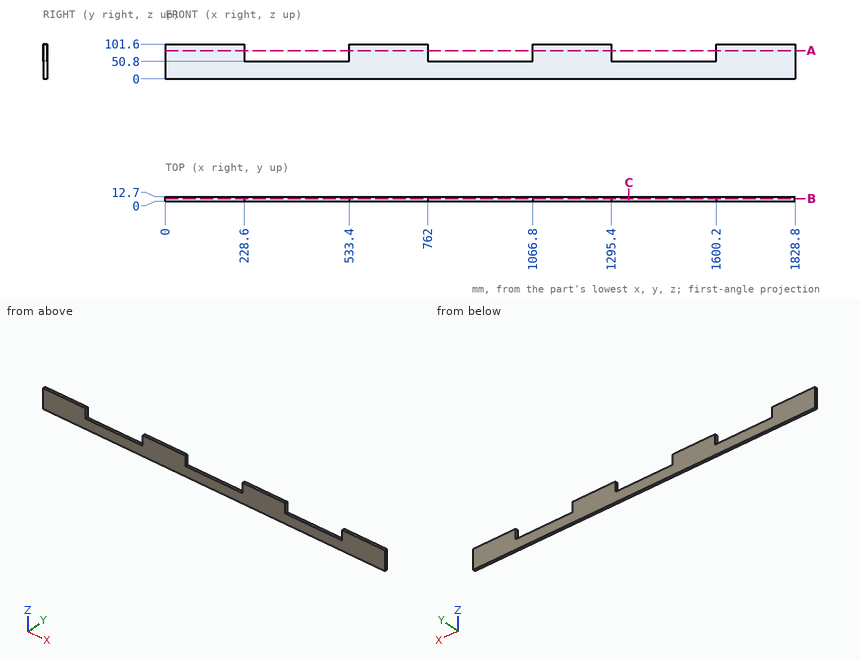
Could you check a few things on this drawing? It's one solid part, dimensions in mm from its lowest x, y, z. Give positions to 0.01 mm unless a question says otherwise; leave off trailing zeros. Write each loop counter-clockwise with the first axis right and the second up, starting at its lowest first coordinate (ties: lowest second). Pieces come first, ordered by that corner, then holes. Notation, with made-up numbers: (8.5, 38) -> (12.5, 38) arc R22 ccw to (12.5, 51) -> close; hole circle Ø5 at (37, 2). An arc over 180 degrees is marked (long way). Answer as CSV lines item,"result". Start each with the question number.
(1) Please list where these lines run through material, in increasing order: line 1 (X direction, y = 11, z = 56); line 2 (Z direction, x = 1585, y = 6.5).
(2) If we section it at A-A, the plane z = 82: Write out the boundary of the cut face in (x, y), and give its area (3 significant figures).
(3) If we section it at C-C, the plane x = 1346: Write out the boundary of the cut face in (y, z), and give its area (3 significant figures).
(4) If we section it at B-B, the plane y = 8.25: Write out the boundary of the cut face in (x, z).
(5) I'm going to push a flat-ended pin straight in: pin 1 Ø4 at (x, y) = (863.5, 6.5) entering from +Z. Where does the tip first touch, or does it pass through?
Answer list:
1,line 1,"0 to 228.6, 533.4 to 762, 1066.8 to 1295.4, 1600.2 to 1828.8"
1,line 2,"0 to 50.8"
2,outline,"(0, 0) -> (228.6, 0) -> (228.6, 12.7) -> (0, 12.7) -> close; (533.4, 0) -> (762, 0) -> (762, 12.7) -> (533.4, 12.7) -> close; (1066.8, 0) -> (1295.4, 0) -> (1295.4, 12.7) -> (1066.8, 12.7) -> close; (1600.2, 0) -> (1828.8, 0) -> (1828.8, 12.7) -> (1600.2, 12.7) -> close"
2,area,"11,600 mm^2"
3,outline,"(0, 0) -> (12.7, 0) -> (12.7, 50.8) -> (0, 50.8) -> close"
3,area,"645 mm^2"
4,outline,"(0, 0) -> (1828.8, 0) -> (1828.8, 101.6) -> (1600.2, 101.6) -> (1600.2, 50.8) -> (1295.4, 50.8) -> (1295.4, 101.6) -> (1066.8, 101.6) -> (1066.8, 50.8) -> (762, 50.8) -> (762, 101.6) -> (533.4, 101.6) -> (533.4, 50.8) -> (228.6, 50.8) -> (228.6, 101.6) -> (0, 101.6) -> close"
5,pin 1,"z = 50.8"
